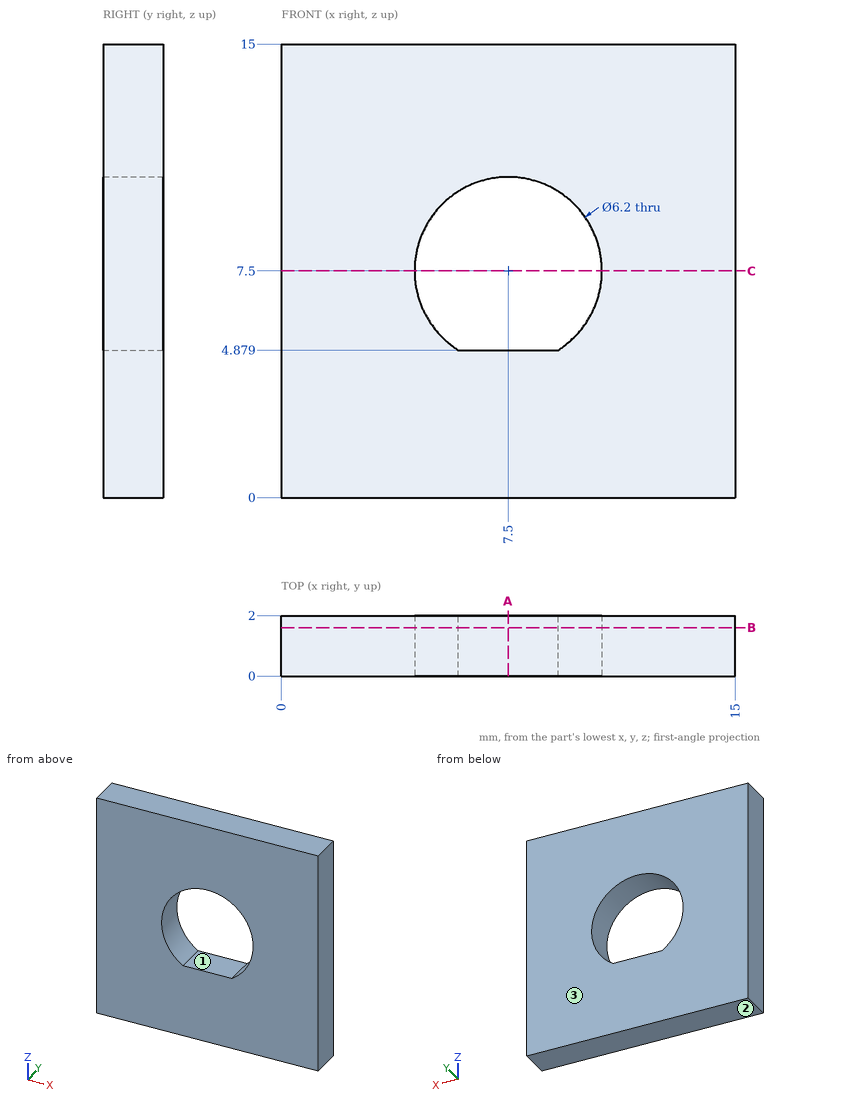
Part print with two shaded views. Sizes in mm from the minimum x, y, z corner. Coordinates: 2 decimals unless noted, no trailing zeros. Order: outer loops, then holes, each group sorted by start corner. A loop starts at its lowest first (then second) coordinate and runs counter-clockwise, first axis right, second up. Notation, with made-up numbers: M 18,3.5 L 70,3.5 A33 cw 70,42.5 Z; hole C 82.25,42 d8. An arc over 180 degrees is marked long. One line per question, with ' | ' between items. Start each with the question number.
1. Mould opens along Z. For the marked faces 1, 2 and 3 say: +Z half, -Z half, draft (parallel to the pull), parting line (faces both ways), or undercut.
2. Flat gauge pin, fed straight in: P1, Ø5, axis at x = 7.5, z = 7.5, coming from the -Y side. Where does the tip first touch, or does it go through?
3. Cut at C-C (z = 7.5). Write the cut outline in (x, y), plus the area to 3 significant figures.
4. Wall check: line 1 along X through (y, z) = (0.85, 7.5); line 2 along Z through (x, y) = (7.5, 0.65); line 3 along X through (y, z) = (0.7, 6.25). Give the ranges that are in metal, low to high. Write a range as [from, to].
5. Cut at A-A (x = 7.5). Write the cut outline in (y, z).
6. Cut at B-B (y = 1.6). Write the cut outline in (x, z) (1 decimal).
The answers:
1) face 1: undercut | face 2: -Z half | face 3: draft
2) P1: passes through
3) outline: M 0,0 L 4.4,0 L 4.4,2 L 0,2 Z; M 10.6,0 L 15,0 L 15,2 L 10.6,2 Z | area: 17.6 mm2
4) line 1: x = [0, 4.4], [10.6, 15] | line 2: z = [0, 4.88], [10.6, 15] | line 3: x = [0, 4.66], [10.34, 15]
5) outline: M 0,0 L 2,0 L 2,4.88 L 0,4.88 Z; M 0,10.6 L 2,10.6 L 2,15 L 0,15 Z
6) outline: M 0,0 L 15,0 L 15,15 L 0,15 Z; hole M 5.8,4.9 L 9.2,4.9 A3.1 ccw long Z
